Verification items for the finished model (mm, model axes). A direction names the side the tool comes from. Coordinates: 2 decimals unless noted, no trailing zeros. Order: outer loops, then holes, each group sorted by start corner. A loop starts at its lowest first (then second) coordinate and runs counter-clockwise, first axis right, second up. Notation, with made-up numbers: M -1,9.25 L 54,9.25 A16 ccw 54,17.25 Z; hole C 21,52 d2. An arc over 180 degrees is marked long. Write item = value, one per line.
```python
from build123d import *

# Parameters (mm, degrees)
F1_DEPTH = 3.175
F2_W     = 25.4
F2_H     = 3.175
F3_DEPTH = 22.225
F4_R     = 2.3114
F5_DEPTH = 25.4
F7_DEPTH = 3.175
F9_DEPTH = 3.175


with BuildPart() as f1:
    # F0 (on Front) → F1 (new body)
    with BuildSketch(Plane.XZ):
        Polygon((-25.4, 0), (0, 0), (0, 28.575), (-25.4, 28.575), (-25.4, 22.225), (-25.4, 3.175), align=None)
        with BuildLine():
            ThreePointArc((-10.3886, 22.225), (-12.7, 19.9136), (-15.0114, 22.225))
            ThreePointArc((-15.0114, 22.225), (-12.7, 24.5364), (-10.3886, 22.225))
        make_face(mode=Mode.SUBTRACT)
    extrude(amount=F1_DEPTH)

    # F2 (on face) → F3 (join)
    with BuildSketch(Plane.XZ.offset(3.175)):
        with Locations((-12.7, 1.5875)):
            Rectangle(F2_W, F2_H)
    extrude(amount=F3_DEPTH)

    # F4 (on face) → F5 (cut)
    with BuildSketch(Plane.XY.offset(3.175)):
        with Locations((-12.7, -19.05)):
            Circle(F4_R)
    extrude(amount=-F5_DEPTH, mode=Mode.SUBTRACT)

    # F6 (on face) → F7 (join)
    with BuildSketch(Plane.YZ):
        Polygon((-3.175, 28.575), (-25.4, 3.175), (-3.175, 3.175), align=None)
    extrude(amount=-F7_DEPTH)

    # F8 (on face) → F9 (join)
    with BuildSketch(Plane(origin=(-25.4, 0, 0), x_dir=(0, -1, 0), z_dir=(-1, 0, 0))):
        Polygon((3.175, 3.175), (25.4, 3.175), (3.175, 28.575), align=None)
    extrude(amount=-F9_DEPTH)


solid = f1.part
```
Item 1: Sectioned sample at B-B, the plane y = -19.05. Enter the section's corners in (x, z) (3 decimals), then the cut area to 3 significant figures.
Report:
outline = M -25.4,0 L -15.011,0 L -15.011,3.175 L -22.225,3.175 L -22.225,10.432 L -25.4,10.432 Z; M -10.389,0 L 0,0 L 0,10.432 L -3.175,10.432 L -3.175,3.175 L -10.389,3.175 Z
area = 112 mm^2
Item 2: Scan lines: L1, parallel to X at y = -12.25, z = 4 (3 decimals); L2, parallel to Z at x = -12.7, y = -2.45 (3 decimals); L3, parallel to Y at x = -12.7, z = 1.9. Record each from-to range of solid material in increasing order. Write a range as from..to.
Report:
L1 = -25.4..-22.225, -3.175..0
L2 = 0..19.914, 24.536..28.575
L3 = -25.4..-21.36, -16.74..0
Item 3: Sectioned sample at D-D, the plane x = -23.5. Enter the section's corners in (y, z) (3 decimals), then the cut area to 3 significant figures.
Report:
outline = M -25.4,0 L 0,0 L 0,28.575 L -3.175,28.575 L -25.4,3.175 Z
area = 444 mm^2
Item 4: Release check for a two-part mould opening along X. For faces 1 (the flat face through (-13, -25.4, 2)), 2 (the flat face through (-13, -14, 3.175)), 3 (the flat face through (0, -10, 11)), 4 (the flat face through (-22.225, -9, 10)) record: pulls with the +X half, pulls with the -X half, needs draft (parallel to the pull), parting line crosses it, or undercut.
Report:
face_1 = needs draft
face_2 = undercut
face_3 = pulls with the +X half
face_4 = undercut
Item 5: Tool access check on faces 5 (the cylindrical face through (-13.767, -1.565, 20.174)), 6 (the flat face through (-3.175, -10, 10)). Record the directions out of +Z, -Z, +X, -X, +Y, -Y that give a thin tool (end or side, any length) a straight path to the whole face; none if there is none.
Report:
face_5 = +Y, -Y
face_6 = +Z, -Y
Item 6: Sectioned sample at A-A, the plane x = -12.7. Enter the section's corners in (y, z) (3 decimals), then the cut area to 3 significant figures.
Report:
outline = M -25.4,0 L -21.361,0 L -21.361,3.175 L -25.4,3.175 Z; M -16.739,0 L 0,0 L 0,19.914 L -3.175,19.914 L -3.175,3.175 L -16.739,3.175 Z; M -3.175,24.536 L 0,24.536 L 0,28.575 L -3.175,28.575 Z
area = 132 mm^2
Item 7: Gauge pin test, flat ends, axial feed: pin 1 (7.5 mm diameter, centred on x = -12.7, y = -19.05, fed in from +Z) (3 decimals); pin 2 (5 mm diameter, centred on x = -18, z = 20, fed in from -Y) (3 decimals); pin 3 (10 mm diameter, centred on x = -22.5, y = -19.5, fed in from +Z). Record the tip position at first contact, or that the pin passes through.
Report:
pin_1 = 3.175
pin_2 = -3.175
pin_3 = 15.63
Item 8: Sectioned sample at C-C, the plane z = 14.75. Enter the section's corners in (x, y) (3 decimals).
Report:
outline = M -25.4,-15.272 L -22.225,-15.272 L -22.225,-3.175 L -3.175,-3.175 L -3.175,-15.272 L 0,-15.272 L 0,0 L -25.4,0 Z
